```python
from build123d import *

# Parameters (mm, degrees)
BOSS_EXTRUDE1_DEPTH     = 17
CUT_EXTRUDE1_DEPTH      = 44
CUT_EXTRUDE1_DEPTH_BACK = 15
SKETCH3_W               = 9.473572921
SKETCH3_H               = 10.746142417
CUT_EXTRUDE4_REACH      = 25.646
SKETCH5_W               = 10
SKETCH5_H               = 10.75
SKETCH6_R               = 4
CUT_EXTRUDE5_DEPTH      = 16.063287133
CUT_EXTRUDE5_DEPTH_BACK = 16.059572792


with BuildPart() as part:
    # Sketch1 → Boss-Extrude1 (new body)
    with BuildSketch(Plane.XY):
        Polygon((-30.543999746, 100.861422718), (-25.501974605, 100.861422718), (-25.501974605, 89.763425291), (-5.459450623, 89.763425291), (-5.459450623, 100.861422718), (-0.421139822, 100.861422718), (-0.421139822, 85.861422718), (-2.179573068, 80.78462442), (-18.874125124, 66.117800283), (-24.336952566, 69.899502921), (-30.543999746, 85.861422718), align=None)
    extrude(amount=BOSS_EXTRUDE1_DEPTH)

    # Sketch2 → Cut-Extrude1 (cut, two sides)
    with BuildSketch(Plane(origin=(-25.501974605, 0, 0), x_dir=(0, 0, -1), z_dir=(1, 0, 0))) as cut_extrude1_sk:
        with BuildLine():
            Line((-17, 100.861422718), (-17, 89.763425291))
            ThreePointArc((-17, 89.763425291), (-14.704510799, 96.659236925), (-8.73400026, 100.803448872))
            Line((-8.73400026, 100.803448872), (-3.73400026, 100.241430104))
            Line((-3.73400026, 100.241430104), (0, 96.527419984))
            Line((0, 96.527419984), (0, 100.861422718))
            Line((0, 100.861422718), (-17, 100.861422718))
        make_face()
    extrude(amount=CUT_EXTRUDE1_DEPTH, mode=Mode.SUBTRACT)
    extrude(cut_extrude1_sk.sketch, amount=-CUT_EXTRUDE1_DEPTH_BACK, mode=Mode.SUBTRACT)

    # Cut-Sweep1: sweep along a path in Sketch4
    with BuildLine(Plane.XY.offset(10)) as cut_sweep1_path:
        Line((-14.80649526, 69.691373965), (-22.116585307, 75.218908697))
    # Sketch3 → Cut-Sweep1 (sweep, cut)
    with BuildSketch(Plane(origin=(-41.005446227, 46.67455955, 0), x_dir=(0.7512574, 0.660009333, 0), z_dir=(0.660009333, -0.7512574, 0))):
        with Locations((38.216319794, 7.888020567)):
            Rectangle(SKETCH3_W, SKETCH3_H)
    sweep(path=cut_sweep1_path.line, mode=Mode.SUBTRACT)

    # Cut-Extrude4: up to this face of the body (flat: up to its plane)
    cut_extrude4_end = Plane(part.part.faces().sort_by_distance((-19.508744094, 71.535131374, 7.888020567))[0])
    # Sketch5 → Cut-Extrude4 (cut, up to the picked face)
    with BuildSketch(Plane(origin=(0, 89.763425291, 0), x_dir=(1, 0, 0), z_dir=(0, 1, 0)), mode=Mode.PRIVATE) as cut_extrude4_sk1:
        with Locations((-17.083999746, -7.885)):
            Rectangle(SKETCH5_W, SKETCH5_H)
    cut_extrude4_tool1 = split(extrude(cut_extrude4_sk1.sketch, amount=-CUT_EXTRUDE4_REACH, mode=Mode.PRIVATE), bisect_by=cut_extrude4_end, keep=Keep.BOTH, mode=Mode.PRIVATE)
    add(cut_extrude4_tool1.solids().sort_by_distance((-17.084, 89.763425, 7.885))[0], mode=Mode.SUBTRACT)

    # Sketch6 → Cut-Extrude5 (cut, two sides)
    with BuildSketch(Plane.ZY.offset(15.480712614)) as cut_extrude5_sk:
        with Locations((8.5, 94.459280843)):
            Circle(SKETCH6_R)
    extrude(amount=CUT_EXTRUDE5_DEPTH, mode=Mode.SUBTRACT)
    extrude(cut_extrude5_sk.sketch, amount=-CUT_EXTRUDE5_DEPTH_BACK, mode=Mode.SUBTRACT)


solid = part.part
```
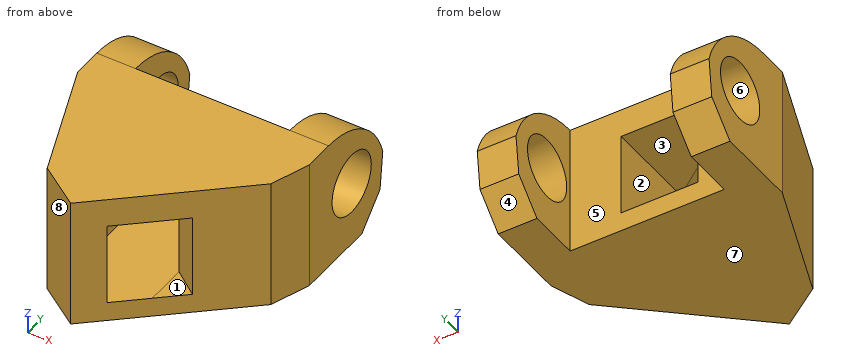
Can you work these out from the model? Positions are in its coordinate system, mm. Face numbers are marked on the shaded views. A direction names the side the tool comes from. Coordinates: 2 decimals unless noted, no trailing zeros. Write each loop counter-clockwise with the first axis right and the second up, starting at its lowest first coordinate (ties: lowest second). Pieces come first, ordered by that corner, then holes. Notation, with made-up numbers: M 6,-29 L 30,-29 A37 ccw 30,8 Z; hole C -29.75,-35.5 d10. An arc over 180 degrees is marked long. Write item = value, one per line. Start each with the question number.
Q1. If we section it at B-B, the plane y = 98: Write out the boundary of the cut face in (x, z), then the cut area to 3 significant figures.
Q2. If I drill on L1, parallel to X at y = 99, z = 11; L2, parallel to Z at x = -17, y = 71; L3, parallel to Y at x = -2.2, z = 8.5, over which ranges is the centre line in solid material (lowest first)? Write a range as [from, to].
Q3. If we section it at A-A, the plane z = 6.5: Write out the boundary of the cut face in (x, y).
Q4. If we section it at C-C, the plane x = -4.5: Write out the boundary of the cut face in (y, z).
Q5. If we section it at D-D, the plane z = 1.5: Write out the boundary of the cut face in (x, y), then the cut area to 3 significant figures.
Q6. On a 3-axis mill with a long thin cutter (end or side, diameter ignored), from which of +Z, -Z, +X, -X, +Y, -Y can I reach the whole of each face in a straight line? I mean the marked faces 1, 2, 3, 4 and 5. Say none if no direction works.
Q7. Thinking about a two-plate mould opening in Z: for the marked faces 6, 7 and 8, which applies, released by +Z, released by -Z, zero draft, split by the parting line, or undercut?
Q8. I'm going to push flat-ended pins straight in: pin 1 (11 mm diameter, centred on x = -14.5, y = 83.5, fed in from -Z); pin 2 (5 mm diameter, centred on y = 82, z = 7, fed in from -X); pin 3 (4 mm diameter, centred on y = 83, z = 3, fed in from -X); pin 4 (5.5 mm diameter, centred on y = 78, z = 6, fed in from -X). Where does each tip first touch, or does it pass through?
Check sheet entries:
q1.outline = M -30.54,1.48 L -25.5,1.48 L -25.5,6.64 L -30.54,6.64 Z; M -30.54,10.36 L -25.5,10.36 L -25.5,13.53 L -30.54,13.53 Z; M -5.46,1.48 L -0.42,1.48 L -0.42,6.64 L -5.46,6.64 Z; M -5.46,10.36 L -0.42,10.36 L -0.42,13.53 L -5.46,13.53 Z
q1.area = 83.9 mm²
q2.L1 = [-30.54, -25.5], [-5.46, -0.42]
q2.L2 = [0, 2.51], [13.26, 17]
q2.L3 = [80.77, 90.46], [98.46, 100.78]
q3.outline = M -30.54,85.86 L -24.34,69.9 L -18.87,66.12 L -15.85,68.77 L -23.16,74.3 L -22.08,75.25 L -22.08,89.76 L -25.5,89.76 L -25.5,91 L -30.54,91 Z; M -30.54,97.92 L -25.5,97.92 L -25.5,100.55 L -30.54,100.55 Z; M -12.08,77.56 L -8.74,75.02 L -2.18,80.78 L -0.42,85.86 L -0.42,91 L -5.46,91 L -5.46,89.76 L -12.08,89.76 Z; M -5.46,97.92 L -0.42,97.92 L -0.42,100.55 L -5.46,100.55 Z
q4.outline = M 78.75,0 L 96.53,0 L 100.24,3.73 L 100.8,8.73 A11.51 ccw 89.76,17 L 78.75,17 Z; hole C 94.46,8.5 d8
q5.outline = M -30.54,85.86 L -24.34,69.9 L -18.87,66.12 L -2.18,80.78 L -0.42,85.86 L -0.42,98.02 L -5.46,98.02 L -5.46,89.76 L -25.5,89.76 L -25.5,98.02 L -30.54,98.02 Z
q5.area = 559 mm²
q6.face_1 = -Y
q6.face_2 = +Y, -Y
q6.face_3 = +Y
q6.face_4 = -Z, +X, -X, +Y
q6.face_5 = +Z, -Z, +Y
q7.face_6 = undercut
q7.face_7 = released by -Z
q7.face_8 = zero draft
q8.pin_1 = 0
q8.pin_2 = -30.01
q8.pin_3 = -30.21
q8.pin_4 = -28.56
